Model file for the job. Use its own axes, mm. Face numbers are marked on the shaded views. A direction names the side the tool comes from. Round coordinates to 2 decimals unless told otherwise and drop trailing zeros. Loops run counter-clockwise (first coordinate to the right, second up) from the corner with the lowest first, then second, coordinate; pieces in that order, holes last.
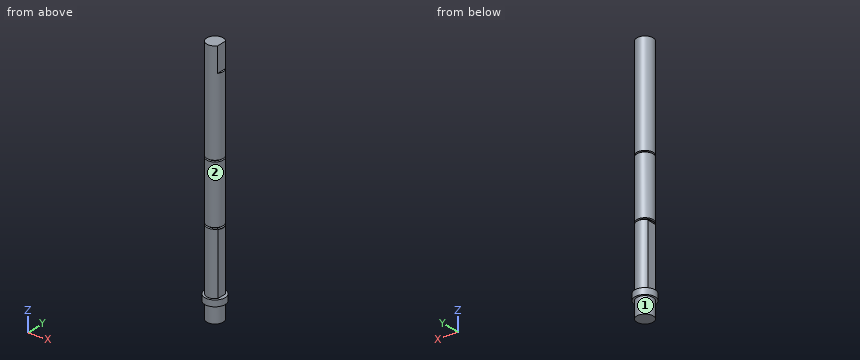
from build123d import *

# Parameters (mm, degrees)
SKETCH1_R           = 4
LOWER_SEAT_DEPTH    = 8
SKETCH2_R           = 5
COLLAR_DEPTH        = 3
SKETCH3_R           = 4
UPPER_DEPTH         = 110
SKETCH4_R           = 5
SKETCH4_R_2         = 3
ECLIP_GROOVE1_DEPTH = 0.74
SKETCH5_R           = 5
SKETCH5_R_2         = 3
ECLIP_GROOVE2_DEPTH = 0.74
SKETCH6_W           = 3
SKETCH6_H           = 10
BURR_FLATS_DEPTH    = 30
SKETCH7_W           = 3
SKETCH7_H           = 10
CRANK_FLAT_DEPTH    = 12


with BuildPart() as part:
    # Sketch1 → Lower_seat (new body)
    with BuildSketch(Plane.XY):
        Circle(SKETCH1_R)
    extrude(amount=LOWER_SEAT_DEPTH)

    # Sketch2 → Collar (add)
    with BuildSketch(Plane.XY.offset(8)):
        Circle(SKETCH2_R)
    extrude(amount=COLLAR_DEPTH)

    # Sketch3 → Upper (add)
    with BuildSketch(Plane.XY.offset(11)):
        Circle(SKETCH3_R)
    extrude(amount=UPPER_DEPTH)

    # Sketch4 → Eclip_groove1 (cut)
    with BuildSketch(Plane.XY.offset(41.2)):
        Circle(SKETCH4_R)
        Circle(SKETCH4_R_2, mode=Mode.SUBTRACT)
    extrude(amount=ECLIP_GROOVE1_DEPTH, mode=Mode.SUBTRACT)

    # Sketch5 → Eclip_groove2 (cut)
    with BuildSketch(Plane.XY.offset(70.5)):
        Circle(SKETCH5_R)
        Circle(SKETCH5_R_2, mode=Mode.SUBTRACT)
    extrude(amount=ECLIP_GROOVE2_DEPTH, mode=Mode.SUBTRACT)

    # Sketch6 → Burr_flats (cut)
    with BuildSketch(Plane.XY.offset(11)):
        with Locations((4.75, 0)):
            Rectangle(SKETCH6_W, SKETCH6_H)
        with Locations((-4.75, 0)):
            Rectangle(SKETCH6_W, SKETCH6_H)
    extrude(amount=BURR_FLATS_DEPTH, mode=Mode.SUBTRACT)

    # Sketch7 → Crank_flat (cut)
    with BuildSketch(Plane.XY.offset(109)):
        with Locations((4.7, 0)):
            Rectangle(SKETCH7_W, SKETCH7_H)
    extrude(amount=CRANK_FLAT_DEPTH, mode=Mode.SUBTRACT)


solid = part.part
Q1. Flat gauge pins, fed straight in: P1, Ø3.5, axis at y = 1, z = 31.5, coming from the -X side; P2, Ø1, axis at x = 0, z = 76.5, coming from the -Y side; P3, Ø3.5, axis at y = 1, z = 32, coming from the +X side. Where does each tip first touch, or does it go through?
Q2. Slice it at D-D on z = 39. Give the cut face in (x, y), plus the area to 3 significant figures.
Q3. Probe line 1 (Z direction, x = 2.25, y = 2.75); line 2 (Z direction, x = 3.75, y = 1); line 3 (Z direction, x = 2.75, y = -4). List the from-to ranges inside material, lowest first.
Q4. Slice it at A-A on x = 0. Give the cut face in (y, z), plus the area to 3 significant figures.
Q5. Tool access for the marked faces 1 and 2: list every direction of +Z, -Z, +X, -X, +Y, -Y with a clear straight run to the whole face (end or side of a thin tool).
Q6. Slice it at C-C on z = 87.5. Give the cut face in (x, y), plus the area to 3 significant figures.
Reply:
1. P1: stops at x = -3.25
1. P2: stops at y = -4
1. P3: stops at x = 3.25
2. outline: (-3.25, -2.33) arc R4 ccw to (3.25, -2.33) - (3.25, 2.33) arc R4 ccw to (-3.25, 2.33) - close
2. area: 45.5 mm2
3. line 1: z = 0 to 41.2, 41.94 to 70.5, 71.24 to 121
3. line 2: z = 0 to 11, 41 to 41.2, 41.94 to 70.5, 71.24 to 109
3. line 3: z = 8 to 11
4. outline: (-5, 8) - (-4, 8) - (-4, 0) - (4, 0) - (4, 8) - (5, 8) - (5, 11) - (4, 11) - (4, 41.2) - (3, 41.2) - (3, 41.94) - (4, 41.94) - (4, 70.5) - (3, 70.5) - (3, 71.24) - (4, 71.24) - (4, 121) - (-4, 121) - (-4, 71.24) - (-3, 71.24) - (-3, 70.5) - (-4, 70.5) - (-4, 41.94) - (-3, 41.94) - (-3, 41.2) - (-4, 41.2) - (-4, 11) - (-5, 11) - close
4. area: 971 mm2
5. face 1: -Z
5. face 2: +Z
6. outline: circle Ø8 at (0, 0)
6. area: 50.3 mm2
